Autodesk Inventor part; units mm, degrees
ref_plane "YZ Plane" through (0, 0, 0) normal (1, 0, 0) x (0, 1, 0)
ref_plane "XZ Plane" through (0, 0, 0) normal (0, 1, 0) x (-1, 0, 0)
ref_plane "XY Plane" through (0, 0, 0) normal (0, 0, 1) x (1, 0, 0)
sketch "Sketch1" plane through (0, 0, 0) normal (0, 0, 1) x (1, 0, 0)
  line L0 (7.65, 0) -> (12.5, 0)
  line L1 (12.5, 0) -> (12.5, 12) construction
  line L2 (12.5, 12) -> (7.65, 12)
  line L3 (7.65, 12) -> (7.65, 0)
  line L4 (0, 0) -> (0, 8.5122) construction
  line L5 (9.5, 9.5) -> (9.5, 2.5)
  line L6 (9.5, 9.5) -> (12, 9.5)
  line L7 (12, 9.5) -> (12.5, 10)
  line L8 (12.5, 0) -> (9.5, 2.5)
  line L9 (12.5, 10) -> (12.5, 12)
  line L10 (7.65, 12) -> (5.65, 12)
  line L11 (5.65, 12) -> (5.65, 9.5)
  line L12 (5.65, 9.5) -> (7.65, 9.5)
  line L13 (7.65, 9.5) -> (7.65, 12)
  point P0 (12.5, 0.6699)
  point P1 (12.5, 6)
  point P2 (15.2143, 7.5754)
  point P3 (15.2143, 2.4246)
  point P4 (9.5, 6)
  point P5 (17.7886, 0.302)
  point P6 (7.65, 6)
  dimension "d6" = 12
  dimension "d7" = 7.65
  dimension "d17" = 7
  dimension "d18" = 2.5
  dimension "d19" = 135
  dimension "d20" = 3
  dimension "d21" = 2
  dimension "d22" = 2.5
  dimension "d23" = 12.5
revolve "Revolution1" add sketch "Sketch1" angle 360 about axis through (0, 0, 0) along (0, 1, 0)
properties part number "pully 15mmx25mmx12mm"
Verification items for the finished model (mm, model axes). A direction names the side the tool comes from. Round coordinates to 2 decimals unless told otherwise and drop trailing zeros. Loops run counter-clockwise (first coordinate to the right, second up) from the corner with the lowest first, then second, coordinate; pieces in that order, holes last. Notation, with made-up numbers: (19.25, -31.5) - (69.25, -31.5) arc R17 cw to (69.25, -12.5) - close; hole circle Ø6 at (5, 26). An arc over 180 degrees is marked (long way). Use a Markdown table: item, result. Add a question column.
1. Gauge pin test, flat ends, axial feed: pin 1 (1.5 mm diameter, centred on x = 0.5, y = 10.5, fed in from -Z); pin 2 (14.5 mm diameter, centred on x = 0, z = 0, fed in from -Y); pin 3 (4 mm diameter, centred on y = 8.5, z = 7, fed in from -X); pin 4 (1 mm diameter, centred on y = 9.5, z = -5, fed in from -X). Record the tip position at first contact, or that the pin passes through.
2. Release check for a two-part mould opening along Z. For faces 4 (the face through (4.38, 5.95, -8.43)), 5 (the face through (-1.658, 4.684, -7.468)), 6 (the face through (-6, 0, 5)) record: released by +Z, released by -Z, zero draft, split by the parting line, or undercut.
3. Section check A-A, the plane z = 0. Record the boundary of the cut face in (x, y).
4. Section check B-B, the plane x = 0. Record the boundary of the cut face in (y, z).
5. Section check C-C, the plane y = 3.5. Record the boundary of the cut face in (x, z), plus the area to 3 significant figures.
6. Access from +Z, -Z, +X, -X, +Y, -Y to the whole of each face (thin tool, end or side, straight path). Record for faces 1 (the face through (9, 9.5, -4)), 2 (the face through (-1, 9.5, 6)), 3 (the face through (11.923, 11.014, -3.755)).
7. Thickness scan on probe 1 along X at (y, z) = (3.75, 0); probe 2 along X at (y, z) = (10, 0). Record the ranges inside material, lowest first. Write a range as [from, to].
Checks:
| question | item | result |
|---|---|---|
| 1 | pin 1 | stops at z = -12.5 |
| 1 | pin 2 | stops at y = 9.5 |
| 1 | pin 3 | stops at x = -11.14 |
| 1 | pin 4 | stops at x = -11.5 |
| 2 | face 4 | split by the parting line |
| 2 | face 5 | undercut |
| 2 | face 6 | zero draft |
| 3 | outline | (-12.5, 0) - (-7.65, 0) - (-7.65, 9.5) - (-5.65, 9.5) - (-5.65, 12) - (-12.5, 12) - (-12.5, 10) - (-12, 9.5) - (-9.5, 9.5) - (-9.5, 2.5) - close; (5.65, 9.5) - (7.65, 9.5) - (7.65, 0) - (12.5, 0) - (9.5, 2.5) - (9.5, 9.5) - (12, 9.5) - (12.5, 10) - (12.5, 12) - (5.65, 12) - close |
| 4 | outline | (0, -12.5) - (2.5, -9.5) - (9.5, -9.5) - (9.5, -12) - (10, -12.5) - (12, -12.5) - (12, -5.65) - (9.5, -5.65) - (9.5, -7.65) - (0, -7.65) - close; (0, 7.65) - (9.5, 7.65) - (9.5, 5.65) - (12, 5.65) - (12, 12.5) - (10, 12.5) - (9.5, 12) - (9.5, 9.5) - (2.5, 9.5) - (0, 12.5) - close |
| 5 | outline | circle Ø19 at (0, 0); hole circle Ø15.3 at (0, 0) |
| 5 | area | 99.7 mm^2 |
| 6 | face 1 | none |
| 6 | face 2 | -Y |
| 6 | face 3 | +Y, -Y |
| 7 | probe 1 | x = [-9.5, -7.65], [7.65, 9.5] |
| 7 | probe 2 | x = [-12.5, -5.65], [5.65, 12.5] |
